For this review, take the finished solid that the model builds, in its own axes (mm). A direction names the side the tool comes from. Round coordinates to 2 decimals unless told otherwise and drop trailing zeros. Loops run counter-clockwise (first coordinate to the right, second up) from the corner with the lowest first, then second, coordinate; pieces in that order, holes last.
1) Take a section at A-A (x = -7). State the section outline as (y, z) points.
2) Mouldability with a two-part tool opening along X and no side actions: class faces 4 (the flat face through (65, 1, 1)), 5 (the flat face through (-65, 1, -55)), 6 (the flat face through (-46.95, 1, -60)), 7 (the flat face through (14, 3, -1)) as pulls with the +X half, pulls with the -X half, needs draft (parallel to the pull), parting line crosses it, or undercut.
3) Insertion check: pin 1 (4 mm diameter, centred on x = 14.24, z = 16, fed in from +Y). The pin has a flat end and moves straight along its axis. Give the tip position at first contact, or say it passes through.
4) Wall thickness on L1, parallel to X at y = 1.05, z = -45.74 (3 decimals); L2, parallel to X at y = 1.45, z = -40 (3 decimals); L3, parallel to Z at x = -37.5, y = 1.1: over which ranges is each line inside the solid? List them lowest first.
5) Take a section at C-C (z = 23.5). State the section outline as (x, y) points.
6) Tool access review of faces 1 (the flat face through (14, 0, -1)), 2 (the flat face through (-35, 1, 35)), 3 (the flat face through (0, 1, -57.5)): name each direction out of +Z, -Z, +X, -X, +Y, -Y from which nothing blocks a thin tool from reaching the whole face with its end or side.
7) Take a section at B-B (y = 2.05). Give the number of separate pieces and of enclosed holes in the cut face, then the cut area to 3 significant figures.
```python
from build123d import *

# Parameters (mm, degrees)
SKETCH1_R           = 1.525
SKETCH1_R_2         = 4.85
SKETCH1_W           = 3.05
SKETCH1_H           = 5
BOSS_EXTRUDE1_DEPTH = 3


with BuildPart() as part:
    # Sketch1 → Boss-Extrude1 (new body)
    with BuildSketch(Plane(origin=(0, 0, 0), x_dir=(1, 0, 0), z_dir=(0, 1, 0))):
        Polygon((-65, -75), (65, -75), (65, -52.5), (65, -47.5), (65, 75), (-65, 75), (-65, 35), (-5, 35), (-5, -35), (-65, -35), (-65, -47.5), (-65, -52.5), align=None)
        with Locations(Location((-61.3, 70, 0), (0, 0, 270))):
            Circle(SKETCH1_R, mode=Mode.SUBTRACT)
        with Locations(Location((-61.3, 45.74, 0), (0, 0, 270))):
            Circle(SKETCH1_R, mode=Mode.SUBTRACT)
        with Locations(Location((-36.5, 70, 0), (0, 0, 270))):
            Circle(SKETCH1_R, mode=Mode.SUBTRACT)
        with Locations(Location((-36.5, 45.74, 0), (0, 0, 270))):
            Circle(SKETCH1_R, mode=Mode.SUBTRACT)
        with Locations(Location((36.5, 45.74, 0), (0, 0, 270))):
            Circle(SKETCH1_R, mode=Mode.SUBTRACT)
        with Locations(Location((36.5, 70, 0), (0, 0, 270))):
            Circle(SKETCH1_R, mode=Mode.SUBTRACT)
        with Locations(Location((61.3, 45.74, 0), (0, 0, 270))):
            Circle(SKETCH1_R, mode=Mode.SUBTRACT)
        with Locations(Location((61.3, 70, 0), (0, 0, 270))):
            Circle(SKETCH1_R, mode=Mode.SUBTRACT)
        with Locations(Location((-47, -70, 0), (0, 0, 270))):
            Circle(SKETCH1_R, mode=Mode.SUBTRACT)
        with Locations(Location((47, -70, 0), (0, 0, 270))):
            Circle(SKETCH1_R, mode=Mode.SUBTRACT)
        with Locations(Location((-60, 40, 0), (0, 0, 270))):
            Circle(SKETCH1_R, mode=Mode.SUBTRACT)
        with Locations(Location((60, 40, 0), (0, 0, 270))):
            Circle(SKETCH1_R, mode=Mode.SUBTRACT)
        with Locations(Location((59, -45, 0), (0, 0, 270))):
            Circle(SKETCH1_R, mode=Mode.SUBTRACT)
        with Locations(Location((4, 8, 0), (0, 0, 270))):
            Circle(SKETCH1_R, mode=Mode.SUBTRACT)
        with Locations(Location((59, 8, 0), (0, 0, 270))):
            Circle(SKETCH1_R, mode=Mode.SUBTRACT)
        with Locations(Location((53, -16, 0), (0, 0, 270))):
            Circle(SKETCH1_R, mode=Mode.SUBTRACT)
        with Locations(Location((14.24, -16, 0), (0, 0, 270))):
            Circle(SKETCH1_R, mode=Mode.SUBTRACT)
        with Locations(Location((-62.5, -68, 0), (0, 0, 270))):
            Circle(SKETCH1_R, mode=Mode.SUBTRACT)
        with Locations(Location((-31.37, -68, 0), (0, 0, 270))):
            Circle(SKETCH1_R, mode=Mode.SUBTRACT)
        with Locations(Location((-20, -65, 0), (0, 0, 270))):
            Circle(SKETCH1_R_2, mode=Mode.SUBTRACT)
        with Locations((48.475, 60)):
            Rectangle(SKETCH1_W, SKETCH1_H, mode=Mode.SUBTRACT)
        with Locations((-48.475, 60)):
            Rectangle(SKETCH1_W, SKETCH1_H, mode=Mode.SUBTRACT)
        with Locations((0, 60)):
            Rectangle(SKETCH1_W, SKETCH1_H, mode=Mode.SUBTRACT)
    extrude(amount=BOSS_EXTRUDE1_DEPTH)


solid = part.part
```
Response:
1. outline: (0, -75) - (3, -75) - (3, -35) - (0, -35) - close; (0, 35) - (3, 35) - (3, 75) - (0, 75) - close
2. face 4: pulls with the +X half
2. face 5: pulls with the -X half
2. face 6: undercut
2. face 7: needs draft
3. pin 1: stops at y = 3
4. L1: x = -65 to -62.825, -59.775 to -38.025, -34.975 to 34.975, 38.025 to 59.775, 62.825 to 65
4. L2: x = -65 to -61.525, -58.475 to 58.475, 61.525 to 65
4. L3: z = -75 to -71.15, -68.85 to -46.89, -44.59 to -35, 35 to 75
5. outline: (-5, 0) - (65, 0) - (65, 3) - (-5, 3) - close
6. face 1: +Z, -Z, +X, -X, -Y
6. face 2: -X, +Y, -Y
6. face 3: +Y, -Y
7. separate pieces: 1
7. enclosed holes: 23
7. area: 15,000 mm2
